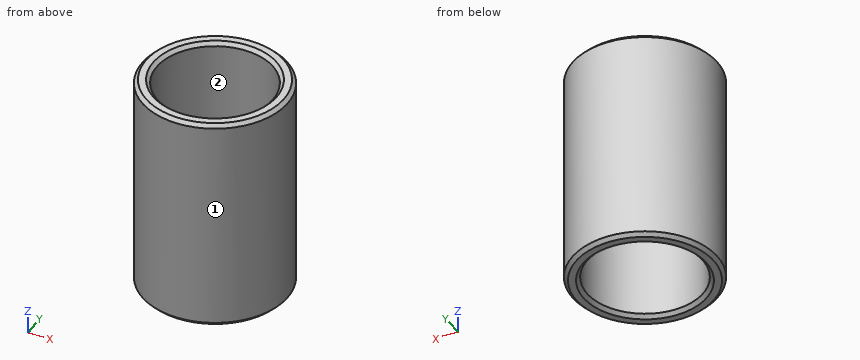
```python
from build123d import *

# Parameters (mm, degrees)
SKETCH_R     = 10
SKETCH_R_2   = 8
PAD_DEPTH    = 30
CHAMFER_SIZE = 0.5


with BuildPart() as part:
    # Sketch → Pad (new body)
    with BuildSketch(Plane.XY):
        Circle(SKETCH_R)
        Circle(SKETCH_R_2, mode=Mode.SUBTRACT)
    extrude(amount=PAD_DEPTH)

    # Chamfer
    chamfer_edges = [part.edges().sort_by_distance(p)[0] for p in [
        (-10, 0, 30),
        (-8, 0, 30),
        (-10, 0, 0),
        (-8, 0, 0),
    ]]
    chamfer(chamfer_edges, length=CHAMFER_SIZE)


solid = part.part
```
CAD build for the part. Positions are in the model's coordinates, mm. Face numbers are marked on the shaded views. Round coordinates to 2 decimals unless told otherwise and drop trailing zeros. Loops run counter-clockwise (first coordinate to the right, second up) from the corner with the lowest first, then second, coordinate; pieces in that order, holes last. Notation, with made-up numbers: M 66,-17.5 L 90,-17.5 A17 cw 90,4.5 Z; hole C 37.5,-36 d3. An arc over 180 degrees is marked long. Use a Markdown table: item, result. Add a question column.
(1) Flat gauge pins, fed straight in: pin 1 (1 mm diameter, centred on y = -1, z = 20.5, fed in from +X); pin 2 (4 mm diameter, centred on y = -5, z = 11.5, fed in from +X); pin 3 (1.5 mm diameter, centred on y = -8, z = 7.5, fed in from +X). Where does each tip first touch, or does it go through?
(2) Cut at A-A (y = 0). Give the cut face in (x, z), and give its area (3 significant figures).
(3) Drill centre lines: line 1 (Y direction, x = 0, z = 12.75); line 2 (X direction, y = -5.5, z = 4.5); line 3 (Y direction, x = -6, z = 23.5). Where is each one in solid material? Low to high.
(4) Cut at C-C (z = 5.5). Give the cut face in (x, y), and give its area (3 significant figures).
(5) Pull direction Y, two halves, no side cores. Call the marked faces 1 and 2: +Y half, -Y half, draft (parallel to the pull), parting line (faces both ways), or undercut.
Geometry says:
| question | item | result |
|---|---|---|
| 1 | pin 1 | stops at x = 9.99 |
| 1 | pin 2 | stops at x = 9.54 |
| 1 | pin 3 | stops at x = 6.89 |
| 2 | outline | M -10,0.5 L -9.5,0 L -8.5,0 L -8,0.5 L -8,29.5 L -8.5,30 L -9.5,30 L -10,29.5 Z; M 8,0.5 L 8.5,0 L 9.5,0 L 10,0.5 L 10,29.5 L 9.5,30 L 8.5,30 L 8,29.5 Z |
| 2 | area | 119 mm² |
| 3 | line 1 | y = -10 to -8, 8 to 10 |
| 3 | line 2 | x = -8.35 to -5.81, 5.81 to 8.35 |
| 3 | line 3 | y = -8 to -5.29, 5.29 to 8 |
| 4 | outline | C 0,0 d20; hole C 0,0 d16 |
| 4 | area | 113 mm² |
| 5 | face 1 | parting line |
| 5 | face 2 | undercut |
